Design review of the part shown in the three views and the two pictorial views. Dimensions are in mm from the part's minimum x, y and z. A direction names the side the tool comes from. Coordinates: 2 decimals unless noted, no trailing zeros. Loops run counter-clockwise (first coordinate to the right, second up) from the corner with the lowest first, then second, coordinate; pieces in that order, holes last. Notation, with made-up numbers: (50.5, 56.5) -> (64.5, 56.5) arc R20 ccw to (64.5, 60.5) -> close; hole circle Ø8 at (66.25, 8.5). An arc over 180 degrees is marked (long way). Answer in a Markdown table with one row per item.
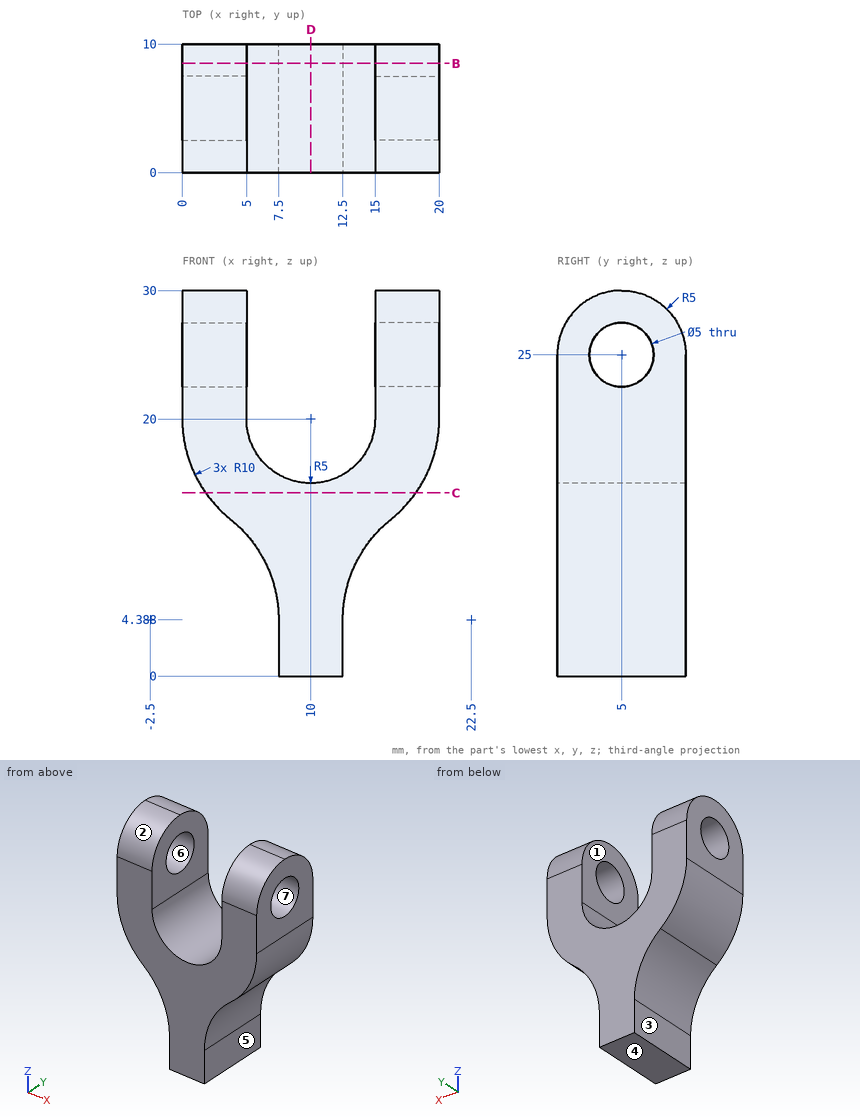
Item 1: Take a section at C-C, the plane z = 14.25. State the section outline as (x, y) points, and give its area (3 significant figures).
Worked answers:
| item | result |
|---|---|
| outline | (1.82, 0) -> (18.18, 0) -> (18.18, 10) -> (1.82, 10) -> close |
| area | 164 mm² |
Item 2: Insertion check: pin 1 (6 mm diameter, centred on y = 2.5, z = 6.5, fed in from +X) (1 decimal); pin 2 (1.3 mm diameter, centred on y = 5, z = 2, fed in from +X); pin 3 (3 mm diameter, centred on y = 6, z = 8, fed in from -X) (1 decimal). Each pin has a flat end and moves straight along its axis. Give the tip position at first contact, or say it passes through.
Worked answers:
| item | result |
|---|---|
| pin 1 | x = 13.9 |
| pin 2 | x = 12.5 |
| pin 3 | x = 6.1 |
Item 3: Take a section at D-D, the plane x = 10. State the section outline as (y, z) points.
Worked answers:
| item | result |
|---|---|
| outline | (0, 0) -> (10, 0) -> (10, 15) -> (0, 15) -> close |
Item 4: The part is to be moulded in two halves that separate along Z. For the marked faces 4, 5, 6 and 7, say which applies: +Z half, -Z half, draft (parallel to the pull), parting line (faces both ways), or undercut.
Worked answers:
| item | result |
|---|---|
| face 4 | -Z half |
| face 5 | draft |
| face 6 | undercut |
| face 7 | undercut |
Item 5: Take a section at B-B, the plane y = 8.5. State the section outline as (x, z) points.
Worked answers:
| item | result |
|---|---|
| outline | (0, 20) arc R10 ccw to (3.75, 12.19) arc R10 cw to (7.5, 4.39) -> (7.5, 0) -> (12.5, 0) -> (12.5, 4.39) arc R10 cw to (16.25, 12.19) arc R10 ccw to (20, 20) -> (20, 28.57) -> (15, 28.57) -> (15, 20) arc R5 cw to (5, 20) -> (5, 28.57) -> (0, 28.57) -> close |
Item 6: For L1, parallel to X at y = 8, z = 24.25; L2, parallel to Y at x = 16.6, z = 25; L3, parallel to X at y = 4.75, z = 4.25, list the stretches that pass through material, from the lowest coordinate up.
Worked answers:
| item | result |
|---|---|
| L1 | 0 to 5, 15 to 20 |
| L2 | 0 to 2.5, 7.5 to 10 |
| L3 | 7.5 to 12.5 |
Item 7: For the marked faces 1, 2 and 3, list the 3-axis set-ups (+Z, -Z, +X, -X, +Y, -Y) from which the entire face can be reached by the end or side of a thin tool; tool diameter is ignored.
Worked answers:
| item | result |
|---|---|
| face 1 | +Z, +Y, -Y |
| face 2 | +Z, +X, -X, -Y |
| face 3 | -Z, -X, +Y, -Y |
